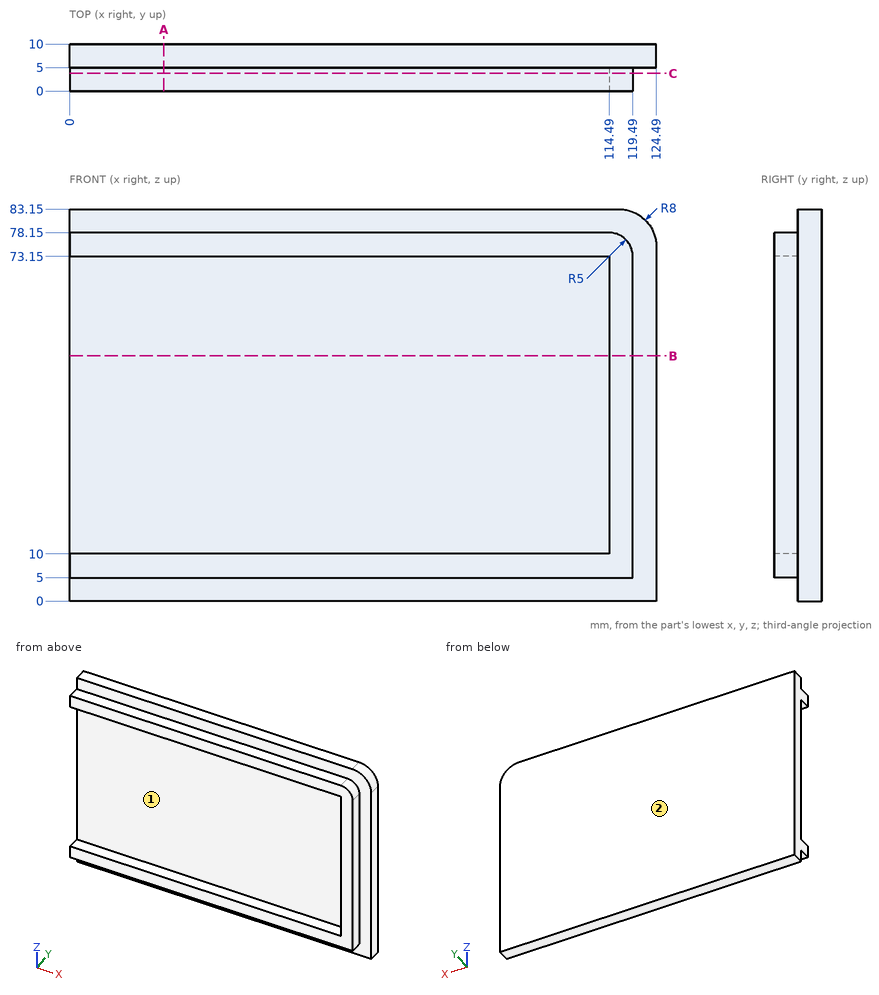
Here's the drawing with two shaded views (mm, measured from the low corner). I have some questions. Round coordinates to 2 decimals unless told otherwise and drop trailing zeros. Order: outer loops, then holes, each group sorted by start corner. A loop starts at its lowest first (then second) coordinate and runs counter-clockwise, first axis right, second up. Notation, with made-up numbers: (2.5, 76.25) -> (12.5, 76.25) arc R19 cw to (12.5, 108.25) -> close; hole circle Ø4 at (46.25, 37). An arc over 180 degrees is marked (long way). Use a Markdown table: item, result. Add a question column.
(1) Suppose I cut it at B-B, the plane z = 52. Please give me the cut outline in (x, y).
(2) I need wall thicknesses on line 1 along Z through (x, y) = (65, 4.25); line 2 along Y through (x, z) = (45.5, 66); line 3 along X through (y, z) = (1.75, 55.5). Which ranges of each line are inside material? Lowest first, please.
(3) Suppose I cut it at C-C, the plane y = 3.75. Please give me the cut outline in (x, z), and give its area (3 significant figures).
(4) Suppose I cut it at A-A, the plane x = 20. Please give me the cut outline in (y, z).
(5) For pin 1 Ø2.5 at (y, z) = (1.5, 40.5) entering from +X; pin 2 Ø1.5 at (x, y) = (35, 3.5) entering from -Z; pin 3 Ø2.5 at (y, z) = (1.5, 33.5) entering from -X, each with a flat end and sliding along its axis, tell me the tip position at first contact or that it passes through.
(6) If we mould it in two halves opening along Z, with no side actions, what happens to the marked faces 1 and 2? For each: released by +Z, released by -Z, zero draft, split by the parting line, or undercut.
Verdict:
| question | item | result |
|---|---|---|
| 1 | outline | (0, 5) -> (114.49, 5) -> (114.49, 0) -> (119.49, 0) -> (119.49, 5) -> (124.49, 5) -> (124.49, 10) -> (0, 10) -> close |
| 2 | line 1 | 5 to 10, 73.15 to 78.15 |
| 2 | line 2 | 5 to 10 |
| 2 | line 3 | 114.49 to 119.49 |
| 3 | outline | (0, 5) -> (119.49, 5) -> (119.49, 73.15) arc R5 ccw to (114.49, 78.15) -> (0, 78.15) -> (0, 73.15) -> (114.49, 73.15) -> (114.49, 10) -> (0, 10) -> close |
| 3 | area | 1,510 mm2 |
| 4 | outline | (0, 5) -> (5, 5) -> (5, 0) -> (10, 0) -> (10, 83.15) -> (5, 83.15) -> (5, 78.15) -> (0, 78.15) -> (0, 73.15) -> (5, 73.15) -> (5, 10) -> (0, 10) -> close |
| 5 | pin 1 | x = 119.49 |
| 5 | pin 2 | z = 5 |
| 5 | pin 3 | x = 114.49 |
| 6 | face 1 | undercut |
| 6 | face 2 | zero draft |
